Geometry check sheet. Reference: the model listing, model coordinates, mm. A direction names the side the tool comes from. Round coordinates to 2 decimals unless told otherwise and drop trailing zeros. Write each loop counter-clockwise with the first axis right and the second up, starting at its lowest first coordinate (ties: lowest second). Pieces come first, ordered by that corner, then holes. Notation, with made-up numbers: (79, 84.25) - (90, 84.25) arc R12 ccw to (90, 91.25) - close; hole circle Ø2 at (-5.75, 48.25). An arc over 180 degrees is marked (long way). One line per question, with ' | ' between items. Start each with the question number.
from build123d import *

# Parameters (mm, degrees)
CROQUIS1_R              = 50
CROQUIS1_R_2            = 45
SALIENTE_EXTRUIR1_DEPTH = 400
CROQUIS2_R              = 55
SALIENTE_EXTRUIR2_DEPTH = 30
SALIENTE_EXTRUIR3_START = -30
CROQUIS3_R              = 55
SALIENTE_EXTRUIR3_DEPTH = 30
CROQUIS5_R              = 12.7
CORTAR_EXTRUIR2_DEPTH   = 60
CROQUIS7_R              = 12.7
CORTAR_EXTRUIR4_DEPTH   = 106


with BuildPart() as part:
    # Croquis1 → Saliente-Extruir1 (new body)
    with BuildSketch(Plane.XY):
        Circle(CROQUIS1_R)
        Circle(CROQUIS1_R_2, mode=Mode.SUBTRACT)
    extrude(amount=SALIENTE_EXTRUIR1_DEPTH)

    # Croquis2 → Saliente-Extruir2 (add)
    with BuildSketch(Plane.XY):
        Circle(CROQUIS2_R)
    extrude(amount=SALIENTE_EXTRUIR2_DEPTH)

    # Croquis3 → Saliente-Extruir3 (add)
    with BuildSketch(Plane.XY.offset(400).offset(SALIENTE_EXTRUIR3_START)):
        Circle(CROQUIS3_R)
    extrude(amount=SALIENTE_EXTRUIR3_DEPTH)

    # Croquis5 → Cortar-Extruir2 (cut)
    with BuildSketch(Plane(origin=(0, 50, 0), x_dir=(1, 0, 0), z_dir=(0, 1, 0))):
        with Locations(Location((0, -350, 0), (0, 0, 270))):
            Circle(CROQUIS5_R)
        with Locations(Location((0, -50, 0), (0, 0, 270))):
            Circle(CROQUIS5_R)
    extrude(amount=-CORTAR_EXTRUIR2_DEPTH, mode=Mode.SUBTRACT)

    # Croquis7 → Cortar-Extruir4 (cut)
    with BuildSketch(Plane(origin=(0, 0, 0), x_dir=(0, 0, -1), z_dir=(1, 0, 0))):
        with Locations(Location((-200, 0, 0), (0, 0, 180))):
            Circle(CROQUIS7_R)
    extrude(amount=-CORTAR_EXTRUIR4_DEPTH, mode=Mode.SUBTRACT)


solid = part.part
Q1. Section check A-A, the plane x = 0. Record the cut outline in (y, z).
Q2. Go/stop test with flat-tipped pins: P1, Ø15, axis at y = 0, z = 200, coming from the -X side; P2, Ø4, axis at x = -2.5, z = 316, coming from the -Y side; P3, Ø8, axis at x = 17.5, z = 230, coming from the -Y side. Record where each tip stops, or that it passes through.
Q3. Section check B-B, the plane x = -18. Record the cut outline in (y, z), then the cut area to 3 significant figures.
Q4. Set-up check for faces 4 (the cylindrical face through (-12.4, 46.63, 347.25)), 5 (the cylindrical face through (-46.538, -10.709, 206.827)), 6 (the flat face through (-1, 1, 30)): record each of +Z, -Z, +X, -X, +Y, -Y from which the full face is reachable in a straight line by a thin tool's end or side.
Q5. Section check D-D, the plane z = 319.5. Record the cut outline in (x, y).
Q6. Draft check along Z on faces 1 (the flat face through (-1, 1, 0)), 2 (the flat face through (-1, 1, 400)), 3 (the flat face through (-1, 1, 370)). Enter one of: pulls with the +Z half, pulls with the -Z half, needs draft (parallel to the pull), parting line crosses it, or undercut.
Q7. Thickness scan on line 1 (Z direction, x = 0, y = 48.75); line 2 (Z direction, x = -44.75, y = 0); line 3 (X direction, y = 0, z = 159). Record the ranges inside material, lowest first.
Q8. Section check C-C, the plane y = 0. Record the cut outline in (x, z).
Result sheet:
1) outline: (-55, 0) - (55, 0) - (55, 30) - (50, 30) - (50, 37.3) - (45, 37.3) - (45, 30) - (-45, 30) - (-45, 370) - (45, 370) - (45, 362.7) - (50, 362.7) - (50, 370) - (55, 370) - (55, 400) - (-55, 400) - (-55, 370) - (-50, 370) - (-50, 30) - (-55, 30) - close; (45, 62.7) - (50, 62.7) - (50, 337.3) - (45, 337.3) - close
2) P1: x = 44.37 | P2: y = -50 | P3: y = -48.14
3) outline: (-51.97, 0) - (51.97, 0) - (51.97, 30) - (46.65, 30) - (46.65, 370) - (51.97, 370) - (51.97, 400) - (-51.97, 400) - (-51.97, 370) - (-46.65, 370) - (-46.65, 30) - (-51.97, 30) - close; hole (-41.24, 30) - (41.24, 30) - (41.24, 370) - (-41.24, 370) - close | area: 9,910 mm²
4) face 4: +Y | face 5: -X | face 6: none
5) outline: circle Ø100 at (0, 0); hole circle Ø90 at (0, 0)
6) face 1: pulls with the -Z half | face 2: pulls with the +Z half | face 3: undercut
7) line 1: 0 to 37.3, 62.7 to 337.3, 362.7 to 400 | line 2: 0 to 30, 370 to 400 | line 3: -50 to -45, 45 to 50
8) outline: (-55, 0) - (55, 0) - (55, 30) - (50, 30) - (50, 370) - (55, 370) - (55, 400) - (-55, 400) - (-55, 370) - (-50, 370) - (-50, 212.7) - (-45, 212.7) - (-45, 370) - (45, 370) - (45, 30) - (-45, 30) - (-45, 187.3) - (-50, 187.3) - (-50, 30) - (-55, 30) - close
